Autodesk Inventor part; units mm, degrees
ref_plane "YZ Plane" through (0, 0, 0) normal (1, 0, 0) x (0, 1, 0)
ref_plane "XZ Plane" through (0, 0, 0) normal (0, 1, 0) x (-1, 0, 0)
ref_plane "XY Plane" through (0, 0, 0) normal (0, 0, 1) x (1, 0, 0)
sketch "Sketch1" plane through (0, 0, 0) normal (0, 1, 0) x (-1, 0, 0)
  line L0 (0, 0) -> (0, 98.75)
  line L1 (0, 98.75) -> (114.73, 98.75)
  line L2 (114.73, 98.75) -> (114.73, 0)
  line L3 (114.73, 0) -> (0, 0)
  line L4 (0, 98.75) -> (0, 90.47)
  line L5 (0, 0) -> (0, 6.72)
  line L6 (114.73, 0) -> (114.73, 9.87)
  line L7 (-2, 0) -> (-2, 98.75)
  line L8 (-2, 98.75) -> (-2, 100.75)
  line L9 (-2, 100.75) -> (114.73, 100.75)
  line L10 (114.73, 100.75) -> (116.73, 100.75)
  line L11 (116.73, 100.75) -> (116.73, 0)
  line L12 (116.73, 0) -> (116.73, -2)
  line L13 (116.73, -2) -> (-2, -2)
  line L14 (-2, -2) -> (-2, 0)
  dimension "d11" = 2
  dimension "d12" = 2
  dimension "d13" = 2
  dimension "d14" = 2
extrude "Extrusion1" add sketch "Sketch1" along normal blind 2 contours L0 L1 L2 L3 | L7 L8 L9 L10 L11 L12 L13 L14
extrude "Extrusion9" add sketch "Sketch1" along normal blind 48
sketch "Sketch11" plane through (0, 2, 0) normal (0, 1, 0) x (1, 0, 0)
  circle A0 centre (-60.73, -74.125) radius 3.75
  line L0 (-68.73, -5.5) -> (-68.73, -51.875)
  line L1 (-68.73, -5.5) -> (-52.73, -5.5)
  line L2 (-68.73, -51.875) -> (-52.73, -51.875)
  line L3 (-52.73, -51.875) -> (-52.73, -5.5)
  line L4 (-68.53, -92.03) -> (-68.53, -66.625)
  line L5 (-68.53, -66.625) -> (-53.65, -66.625)
  line L6 (-53.65, -66.625) -> (-53.65, -92.03)
  line L7 (-53.65, -92.03) -> (-45.73, -92.03)
  line L8 (-45.73, -92.03) -> (-45.73, -5.5)
  line L9 (-48.73, -5.5) -> (-45.73, -5.5)
  line L10 (-48.73, -5.5) -> (-48.73, -55.875)
  line L11 (-48.73, -55.875) -> (-72.73, -55.875)
  line L12 (-72.73, -55.875) -> (-72.73, -5.5)
  line L13 (-75.73, -5.5) -> (-72.73, -5.5)
  line L14 (-75.73, -5.5) -> (-75.73, -17.875)
  line L15 (-75.73, -17.875) -> (-85.89, -17.875)
  line L16 (-85.89, -17.875) -> (-85.89, -5.5)
  line L17 (-85.89, -5.5) -> (-93.51, -5.5)
  line L18 (-93.51, -5.5) -> (-93.51, -17.875)
  line L19 (-93.51, -17.875) -> (-103.67, -17.875)
  line L20 (-103.67, -17.875) -> (-103.67, -5.5)
  line L21 (-111.73, -5.5) -> (-103.67, -5.5)
  line L22 (-111.73, -5.5) -> (-111.73, -93.25)
  line L23 (-111.73, -93.25) -> (-103.67, -93.25)
  line L24 (-103.67, -93.25) -> (-103.67, -80.875)
  line L25 (-103.67, -80.875) -> (-93.51, -80.875)
  line L26 (-93.51, -80.875) -> (-93.51, -92.03)
  line L27 (-93.51, -92.03) -> (-85.89, -92.03)
  line L28 (-85.89, -92.03) -> (-85.89, -80.875)
  line L29 (-85.89, -80.875) -> (-75.73, -80.875)
  line L30 (-75.73, -80.875) -> (-75.73, -92.03)
  line L31 (-75.73, -92.03) -> (-68.53, -92.03)
  line L32 (-56.73, -92.03) -> (-56.73, -81.625)
  line L33 (-56.73, -81.625) -> (-64.73, -81.625)
  line L34 (-64.73, -81.625) -> (-64.73, -92.03)
  line L35 (-64.73, -92.03) -> (-56.73, -92.03)
  circle A1 centre (-98.59, -84.875) radius 1.65
  circle A2 centre (-80.81, -84.875) radius 1.65
  circle A3 centre (-60.73, -74.125) radius 3.75
  line L36 (-114.73, -98.25) -> (-114.73, -0.5)
  line L37 (-114.73, -0.5) -> (-42.73, -0.5)
  line L38 (-42.73, -0.5) -> (-42.73, -98.25)
  line L39 (-114.73, -98.25) -> (-42.73, -98.25)
  circle A4 centre (-70.73, -23.875) radius 1
  circle A5 centre (-50.73, -23.875) radius 1
  circle A6 centre (-60.73, -53.875) radius 1
  circle A7 centre (-80.81, -13.875) radius 1.65
  circle A8 centre (-98.59, -13.875) radius 1.65
  line L40 (-68.73, -5.5) -> (-68.73, -51.875)
  line L41 (-68.73, -51.875) -> (-52.73, -51.875)
  line L42 (-52.73, -51.875) -> (-52.73, -5.5)
  line L43 (-68.73, -5.5) -> (-52.73, -5.5)
  circle A9 centre (-60.73, -74.125) radius 7.5
  line L44 (-67.83, -47.875) -> (-53.63, -47.875)
  line L45 (-67.83, -16.5) -> (-67.83, -47.875)
  line L46 (-53.63, -47.875) -> (-53.63, -16.5)
  line L47 (-53.63, -16.5) -> (-67.83, -16.5)
  line L48 (-42.73, -98.25) -> (-39.73, -98.25)
  line L49 (-39.73, -98.25) -> (-39.73, -0.5)
  line L50 (-39.73, -0.5) -> (-42.73, -0.5)
  line L51 (-42.73, -0.5) -> (-42.73, -98.25)
  circle A10 centre (-96.54, -74.125) radius 3.25
  circle A11 centre (-84.58, -61.395) radius 2.75
  circle A12 centre (-94.53, -61.295) radius 2.75
  circle A13 centre (-94.53, -51.135) radius 2.75
  circle A14 centre (-84.58, -51.395) radius 2.75
  circle A15 centre (-94.53, -40.055) radius 2.75
  circle A16 centre (-84.58, -40.145) radius 2.75
  line L52 (-76.36, -32.405) -> (-103.04, -32.405)
  line L53 (-76.36, -32.405) -> (-76.36, -20.965)
  line L54 (-76.36, -20.965) -> (-103.04, -20.965)
  line L55 (-103.04, -20.965) -> (-103.04, -32.405)
  circle A17 centre (-98.59, -84.875) radius 3
  circle A18 centre (-80.81, -84.875) radius 3
  circle A19 centre (-98.59, -13.875) radius 3
  circle A20 centre (-80.81, -13.875) radius 3
  circle A21 centre (-82.79, -74.125) radius 3.25
  point P0 (0, 0)
  dimension "d49" = 15
  dimension "d56" = 3
  dimension "d109" = 11.44
  dimension "d127" = 6
  dimension "d128" = 6
  dimension "d129" = 6
  dimension "d130" = 6
  dimension "d191" = 6.5
extrude "Extrusion10" cut sketch "Sketch11" against normal blind 10 contours A0 | A9 L6 | A9 L6 | L45 L47 L46 L44
extrude "Extrusion11" add sketch "Sketch11" along normal blind 7 contours L38 L50 L49 L48
sketch "Sketch12" plane through (-42.73, 2, 0.5) normal (-1, 0, 0) x (0, 0, 1)
  line L0 (97.75, 7) -> (97.75, 5)
  line L1 (97.75, 0) -> (97.75, 7)
  line L2 (97.75, 7) -> (0, 7)
  line L3 (0, 7) -> (0, 5)
  line L4 (0, 0) -> (0, 7)
  line L5 (0, 5) -> (97.75, 5)
  line L6 (97.75, 7) -> (0, 7)
  point P0 (-0.5, -2)
  dimension "d61" = 2
  dimension "d62" = 2
extrude "Extrusion12" add sketch "Sketch12" along normal blind 2
extrude "Extrusion13" cut sketch "Sketch11" against normal blind 5 contours A1 | A2 | A7 | A8 | A10 | A11 | A12 | A13 | A14 | A15 | A16 | A21
extrude "Extrusion14" cut sketch "Sketch11" against normal blind 5 contours L52 L55 L54 L53
sketch "Sketch13" plane through (2, 0, 100.75) normal (1, 0, 0) x (0, 0, -1)
  line L0 (88.25, 41) -> (88.75, 41)
  line L1 (88.75, 41) -> (88.75, 48)
  line L2 (88.75, 48) -> (74.75, 48)
  line L3 (74.75, 48) -> (74.75, 41)
  line L4 (74.75, 41) -> (74.75, 30)
  line L5 (74.75, 30) -> (88.5, 30)
  line L6 (88.5, 30) -> (88.75, 30)
  line L7 (88.75, 30) -> (88.75, 41)
  point P0 (100.75, 0)
  point P1 (102.75, 48)
  dimension "d116" = 0.5
  dimension "d118" = 11
extrude "Extrusion15" cut sketch "Sketch13" against normal blind 5
sketch "Sketch14" plane through (-116.73, 0, 100.75) normal (0, 0, 1) x (1, 0, 0)
  line L0 (0, 0) -> (0, 48)
  line L1 (0, 48) -> (2, 48)
  line L2 (2, 48) -> (36, 48)
  line L3 (2, 48) -> (116.73, 48)
  line L4 (36, 48) -> (45, 48)
  line L5 (36, 48) -> (36.715, 48)
  line L6 (0, 48) -> (118.73, 48)
  line L7 (36.715, 48) -> (36.715, 35)
  line L8 (45, 48) -> (45.715, 48)
  line L9 (45.715, 48) -> (45.715, 35)
  line L10 (45.715, 35) -> (45, 35)
  line L11 (36.715, 35) -> (45, 35)
  point P0 (116.73, 0)
  dimension "d121" = 2
  dimension "d122" = 34
  dimension "d123" = 9
  dimension "d124" = 13
  dimension "d196" = 0.715
  dimension "d197" = 0.715
extrude "Extrusion16" cut sketch "Sketch14" against normal blind 120
extrude "Extrusion17" add sketch "Sketch11" along normal blind 2 contours A17 | A18 | A19 | A20
sketch "Sketch15" plane through (0, 0, 0) normal (0, -1, 0) x (1, 0, 0)
  line L0 (-2, 12) -> (-2, 26)
  line L1 (-2, 26) -> (-12, 26)
  line L2 (-12, 26) -> (-12, 12)
  line L3 (-12, 12) -> (-2, 12)
  point P0 (0, 0)
  point P1 (2, 12)
  dimension "d134" = 10
extrude "Extrusion18" cut sketch "Sketch15" against normal blind 0.5
sketch "Sketch16" plane through (-116.73, 0, -2) normal (-1, 0, 0) x (0, 0, 1)
  line L0 (2, 48) -> (0, 48)
  line L1 (0, 48) -> (20, 48)
  line L2 (100.75, 48) -> (2, 48)
  line L3 (20, 48) -> (20, 43)
  line L4 (20, 43) -> (30, 43)
  line L5 (30, 43) -> (25, 43)
  circle A0 centre (25, 43) radius 1.45
  line L6 (102.75, 48) -> (82.75, 48)
  line L7 (28, 48) -> (100.75, 48)
  line L8 (82.75, 48) -> (82.75, 43)
  line L9 (82.75, 43) -> (77.75, 43)
  circle A1 centre (77.75, 43) radius 1.45
  point P0 (2, 0)
  dimension "d137" = 20
  dimension "d138" = 5
  dimension "d139" = 10
  dimension "d140" = 2.9
  dimension "d141" = 20
  dimension "d142" = 5
  dimension "d143" = 5
  dimension "d144" = 2.9
extrude "Extrusion19" cut sketch "Sketch16" against normal blind 3
sketch "Sketch17" plane through (2, 0, 100.75) normal (1, 0, 0) x (0, 0, -1)
  circle A0 centre (51.375, 43) radius 1.45
  point P0 (100.75, 0)
  point P1 (0, 48)
extrude "Extrusion20" cut sketch "Sketch17" against normal blind 3
sketch "Sketch18" plane through (0, 0, 0) normal (0, -1, 0) x (1, 0, 0)
  line L0 (-99.53, 40.055) -> (-99.53, 61.295)
  line L1 (-99.53, 61.295) -> (-99.53, 63.795)
  line L2 (-99.53, 63.795) -> (-103.53, 63.795)
  line L3 (-103.53, 63.795) -> (-103.53, 40.055)
  line L4 (-103.53, 40.055) -> (-103.53, 37.555)
  line L5 (-103.53, 37.555) -> (-99.53, 37.555)
  line L6 (-99.53, 37.555) -> (-99.53, 40.055)
  line L7 (-79.58, 61.395) -> (-79.58, 63.895)
  line L8 (-79.58, 63.895) -> (-75.58, 63.895)
  line L9 (-75.58, 63.895) -> (-75.58, 40.055)
  line L10 (-75.58, 40.055) -> (-75.58, 37.555)
  line L11 (-75.58, 37.555) -> (-79.58, 37.555)
  line L12 (-79.58, 37.555) -> (-79.58, 63.895)
  line L13 (-103.04, 20.965) -> (-76.36, 20.965)
  line L14 (-103.04, 20.965) -> (-105.04, 20.965)
  line L15 (-105.04, 20.965) -> (-105.04, 32.405)
  line L16 (-103.04, 32.405) -> (-76.36, 32.405)
  line L17 (-105.04, 32.405) -> (-109.04, 32.405)
  line L18 (-109.04, 32.405) -> (-109.04, 20.965)
  line L19 (-109.04, 20.965) -> (-105.04, 20.965)
  circle A0 centre (-96.54, 74.125) radius 3.25
  line L20 (-96.54, 74.125) -> (-101.54, 74.125)
  line L21 (-101.54, 74.125) -> (-101.54, 78.125)
  line L22 (-101.54, 78.125) -> (-105.54, 78.125)
  line L23 (-105.54, 78.125) -> (-105.54, 70.125)
  line L24 (-105.54, 70.125) -> (-101.54, 70.125)
  line L25 (-101.54, 70.125) -> (-101.54, 74.125)
  line L26 (-70.73, 74.125) -> (-70.73, 78.125)
  line L27 (-70.73, 78.125) -> (-74.73, 78.125)
  line L28 (-74.73, 78.125) -> (-74.73, 70.125)
  line L29 (-74.73, 70.125) -> (-70.73, 70.125)
  line L30 (-70.73, 74.125) -> (-70.73, 70.125)
  line L31 (-69.83, 47.875) -> (-69.83, 16.5)
  line L32 (-69.83, 16.5) -> (-73.83, 16.5)
  line L33 (-73.83, 16.5) -> (-73.83, 47.875)
  line L34 (-73.83, 47.875) -> (-69.83, 47.875)
  circle A1 centre (-82.79, 74.125) radius 3.25
  line L35 (-82.79, 74.125) -> (-87.79, 74.125)
  line L36 (-87.79, 74.125) -> (-87.79, 78.125)
  line L37 (-87.79, 78.125) -> (-91.79, 78.125)
  line L38 (-91.79, 78.125) -> (-91.79, 70.125)
  line L39 (-91.79, 70.125) -> (-87.79, 70.125)
  line L40 (-87.79, 70.125) -> (-87.79, 74.125)
  point P0 (0, 0)
  point P1 (-94.53, 40.055)
  point P2 (-84.58, 61.395)
  point P3 (-85.81, 74.125)
  point P4 (-85.81, 78.125)
  point P5 (-89.81, 78.125)
  point P6 (-89.81, 70.125)
  point P7 (-85.81, 70.125)
  point P8 (-67.83, 47.875)
  dimension "d153" = 2.5
  dimension "d154" = 4
  dimension "d155" = 2.5
  dimension "d157" = 2.5
  dimension "d158" = 4
  dimension "d159" = 2.5
  dimension "d160" = 4
  dimension "d161" = 2
  dimension "d162" = 4
  dimension "d163" = 5
  dimension "d164" = 4
  dimension "d165" = 4
  dimension "d166" = 8
  dimension "d171" = 4
  dimension "d172" = 4
  dimension "d173" = 8
  dimension "d175" = 4
  dimension "d198" = 5
  dimension "d199" = 4
  dimension "d200" = 8
extrude "Extrusion21" cut sketch "Sketch18" against normal blind 0.5 contours L6 L5 L4 L3 L2 L1 L0 | L7 L8 L9 L10 L11 L12 | L19 L18 L17 L15 | A0 | L25 L24 L23 L22 L21 | L30 L29 L28 L27 L26 | L31 L32 L33 L34 | L40 L39 L38 L37 L36
sketch "Sketch19" plane through (0, 0, 0) normal (0, -1, 0) x (1, 0, 0)
  line L0 (-116.73, -2) -> (2, -2)
  line L1 (2, -2) -> (2, 8)
  line L2 (2, -2) -> (2, 100.75)
  line L3 (2, 8) -> (-18, 8)
  line L4 (2, 100.75) -> (2, 90.75)
  line L5 (2, 90.75) -> (-18, 90.75)
  line L6 (-18, 90.75) -> (-18, 8)
  line L7 (-18, 8) -> (-43, 8)
  line L8 (-43, 8) -> (-43, 90.75)
  line L9 (-43, 90.75) -> (-18, 90.75)
  point P0 (0, 0)
  dimension "d178" = 10
  dimension "d179" = 20
  dimension "d180" = 10
  dimension "d181" = 20
  dimension "d182" = 25
extrude "Extrusion22" cut sketch "Sketch19" against normal blind 0.5 contours L7 L8 L9 L6
fillet "Fillet1" radius 2 1 edges at (-116.73, 0, 49.375)
sketch "Sketch20" plane through (-116.73, 48, -2) normal (-1, 0, 0) x (0, 0, 1)
  line L0 (100.75, 0) -> (2, 0)
  circle A0 centre (51.375, -25) radius 5
  point P0 (2, -48)
  dimension "d187" = 10
extrude "Extrusion23" cut sketch "Sketch20" against normal blind 5
sketch "Sketch21" plane through (0, 0, 0) normal (0, -1, 0) x (1, 0, 0)
  circle A0 centre (-98.59, 13.875) radius 1.65
  circle A1 centre (-98.59, 13.875) radius 3
  circle A2 centre (-80.81, 13.875) radius 1.65
  circle A3 centre (-80.81, 13.875) radius 3
  circle A4 centre (-80.81, 84.875) radius 3
  circle A5 centre (-80.81, 84.875) radius 3
  circle A6 centre (-98.59, 84.875) radius 1.65
  circle A7 centre (-98.59, 84.875) radius 3
  point P0 (0, 0)
  dimension "d201" = 6
  dimension "d202" = 6
  dimension "d203" = 6
  dimension "d204" = 6
extrude "Extrusion24" cut sketch "Sketch21" against normal blind 10
properties part number "case"
Geometry: final body of the model. Coordinates: model frame, mm. A direction names the side the tool comes from. Give positions to 0.01 mm unless a question says otherwise; leave off trailing zeros. Order: outer loops, then holes, each group sorted by start corner. A loop starts at its lowest first (then second) coordinate and runs counter-clockwise, first axis right, second up. Notation, with made-up numbers: (42.25, 81.5) -> (62.25, 81.5) arc R23 cw to (62.25, 116.5) -> close; hole circle Ø2 at (-21.5, -18). An arc over 180 degrees is marked (long way). Write each question's results on one line, items separated by ' | '.
1) Set-up query: faces 3 (the face through (-72, 0.5, 32)), 4 (the face through (-42.73, 4, 49)), 5 (the face through (-42, 6, 98.25)). Return all of +Z, -Z, +X, -X, +Y, -Y with unobstructed straight access to the full face (end or side cutting, diameter ignored); none if empty.
Geometry says:
face 3: -Y | face 4: none | face 5: +Y
2) Cut plane A-A (y = 43). Give the number of separate pieces and of enclosed holes in the cut face, and give its area (3 significant figures).
Geometry says:
separate pieces: 6 | enclosed holes: 0 | area: 789 mm²
3) Line query: line 1 along X through (y, z) = (6, 79.5); line 2 along Z through (x, y) = (-56, 4); line 3 along X through (y, z) = (16, 28). Output: solid intervals per line, ascending.
Geometry says:
line 1: x = -116.73 to -114.73, -42.73 to -39.73, 0 to 2 | line 2: z = -2 to 0, 98.75 to 100.75 | line 3: x = -116.73 to -114.73, 0 to 2
4) Cut plane B-B (y = 5.5). Output: boundary loops of the cut face in (x, z).
Geometry says:
outline: (-116.73, -2) -> (2, -2) -> (2, 100.75) -> (-116.73, 100.75) -> close; (-42.73, 0.5) -> (-39.73, 0.5) -> (-39.73, 98.25) -> (-42.73, 98.25) -> close; hole (-114.73, 0) -> (0, 0) -> (0, 98.75) -> (-114.73, 98.75) -> close
5) Cut plane D-D (z = 92.5). Output: boundary loops of the cut face in (x, y), and give its area (3 significant figures).
Geometry says:
outline: (-116.73, 2) arc R2 ccw to (-114.73, 0) -> (2, 0) -> (2, 48) -> (0, 48) -> (0, 2) -> (-39.73, 2) -> (-39.73, 9) -> (-44.73, 9) -> (-44.73, 7) -> (-42.73, 7) -> (-42.73, 2) -> (-114.73, 2) -> (-114.73, 48) -> (-116.73, 48) -> close | area: 446 mm²
6) First-contact query: pin 1 Ø8 at (x, z) = (-45, 61) entering from +Y; pin 2 Ø2 at (x, z) = (1.5, 17.5) entering from +Y; pin 3 Ø5 at (x, z) = (-35.5, 79) entering from -Y. Flat tips, straight axial feed; report the tip coordinate or a pass-through.
Geometry says:
pin 1: stops at y = 9 | pin 2: stops at y = 30 | pin 3: stops at y = 0.5
7) Draft query along Z for faces 1 (the face through (-28.9, 48, -0.2)), 2 (the face through (-91.99, 1.01, 52.19)). Return one class per face: released by +Z, released by -Z, zero draft, split by the parting line, or undercut.
Geometry says:
face 1: zero draft | face 2: undercut
8) Cut plane C-C (x = -57). Output: boundary loops of the cut face in (y, z) (3 decimals).
Geometry says:
outline: (0, -2) -> (48, -2) -> (48, 0) -> (2, 0) -> (2, 16.5) -> (0, 16.5) -> close; (0, 47.875) -> (2, 47.875) -> (2, 67.618) -> (0, 67.618) -> close; (0, 80.632) -> (2, 80.632) -> (2, 98.75) -> (48, 98.75) -> (48, 100.75) -> (0, 100.75) -> close
